The model under review builds one solid part; all positions refer to its coordinate system, in mm. Coordinates: 2 decimals unless noted, no trailing zeros. Put each result on its own line as item: value. Start each with the question number.
Item 1: For pin 1 (0.7 mm diameter, centred on x = -3.87, y = 1.64, fed in from -Z); pin 2 (1.5 mm diameter, centred on x = -3.5, z = 1, fed in from +Y), all flat-tipped, find the tip position at first contact; note any pin that passes through.
Item 2: Consider section A-A on z = 1.65. State how many separate pieces and enclosed holes the cut face has, then the cut area to 3 significant figures.
Item 3: Mouldability with a two-part tool opening along Y and no side actions: class faces 1 (the face through (-23.977, 1.055, 2.972)), 2 (the face through (7.6, 2.3, 2.5)), 3 (the face through (-4.504, 4.555, 2.465)) as pulls with the +Y half, pulls with the -Y half, needs draft (parallel to the pull), parting line crosses it, or undercut.
Item 4: To check wall thickness, follow L1, parallel to X at y = -1.5, z = 3.6; L2, parallel to X at y = -5.5, z = 0.6; L3, parallel to Y at x = -2.5, z = 1.5. State the ranges of each line that lie inside material, in increasing order. Write a range as [from, to].
```python
from build123d import *

# Parameters (mm, degrees)
SCHIZZO1_R                   = 24
SCHIZZO1_R_2                 = 0.6
ESTRUSIONE_ESTRUSIONE1_DEPTH = 5
SMUSSO1_SIZE                 = 1


with BuildPart() as part:
    # Schizzo1 → Estrusione-Estrusione1 (new body)
    with BuildSketch(Plane.XY):
        Circle(SCHIZZO1_R)
        with Locations((-2.2, 0)):
            Circle(SCHIZZO1_R_2, mode=Mode.SUBTRACT)
        Circle(SCHIZZO1_R_2, mode=Mode.SUBTRACT)
        with Locations((-3.866120385, 1.64107074)):
            Circle(SCHIZZO1_R_2, mode=Mode.SUBTRACT)
        with Locations((-1.1, 1.905255888)):
            Circle(SCHIZZO1_R_2, mode=Mode.SUBTRACT)
        with Locations((1.1, 1.905255888)):
            Circle(SCHIZZO1_R_2, mode=Mode.SUBTRACT)
        with Locations((2.2, 0)):
            Circle(SCHIZZO1_R_2, mode=Mode.SUBTRACT)
        with Locations((1.1, -1.905255888)):
            Circle(SCHIZZO1_R_2, mode=Mode.SUBTRACT)
        with Locations((-1.1, -1.905255888)):
            Circle(SCHIZZO1_R_2, mode=Mode.SUBTRACT)
        with Locations((-2.527623097, 3.354269142)):
            Circle(SCHIZZO1_R_2, mode=Mode.SUBTRACT)
        with Locations((-0.511851242, 4.168693837)):
            Circle(SCHIZZO1_R_2, mode=Mode.SUBTRACT)
        with Locations((1.64107074, 3.866120385)):
            Circle(SCHIZZO1_R_2, mode=Mode.SUBTRACT)
        with Locations((3.354269142, 2.527623097)):
            Circle(SCHIZZO1_R_2, mode=Mode.SUBTRACT)
        with Locations((4.168693837, 0.511851242)):
            Circle(SCHIZZO1_R_2, mode=Mode.SUBTRACT)
        with Locations((3.866120385, -1.64107074)):
            Circle(SCHIZZO1_R_2, mode=Mode.SUBTRACT)
        with Locations((2.527623097, -3.354269142)):
            Circle(SCHIZZO1_R_2, mode=Mode.SUBTRACT)
        with Locations((0.511851242, -4.168693837)):
            Circle(SCHIZZO1_R_2, mode=Mode.SUBTRACT)
        with Locations((-1.64107074, -3.866120385)):
            Circle(SCHIZZO1_R_2, mode=Mode.SUBTRACT)
        with Locations((-3.354269142, -2.527623097)):
            Circle(SCHIZZO1_R_2, mode=Mode.SUBTRACT)
        with Locations((-4.168693837, -0.511851242)):
            Circle(SCHIZZO1_R_2, mode=Mode.SUBTRACT)
        with Locations((-6.3, 0)):
            Circle(SCHIZZO1_R_2, mode=Mode.SUBTRACT)
        with Locations((-5.920063511, 2.154726903)):
            Circle(SCHIZZO1_R_2, mode=Mode.SUBTRACT)
        with Locations((-4.826079992, 4.049561941)):
            Circle(SCHIZZO1_R_2, mode=Mode.SUBTRACT)
        with Locations((-3.15, 5.455960044)):
            Circle(SCHIZZO1_R_2, mode=Mode.SUBTRACT)
        with Locations((-1.093983519, 6.204288844)):
            Circle(SCHIZZO1_R_2, mode=Mode.SUBTRACT)
        with Locations((1.093983519, 6.204288844)):
            Circle(SCHIZZO1_R_2, mode=Mode.SUBTRACT)
        with Locations((3.15, 5.455960044)):
            Circle(SCHIZZO1_R_2, mode=Mode.SUBTRACT)
        with Locations((4.826079992, 4.049561941)):
            Circle(SCHIZZO1_R_2, mode=Mode.SUBTRACT)
        with Locations((5.920063511, 2.154726903)):
            Circle(SCHIZZO1_R_2, mode=Mode.SUBTRACT)
        with Locations((6.3, 0)):
            Circle(SCHIZZO1_R_2, mode=Mode.SUBTRACT)
        with Locations((5.920063511, -2.154726903)):
            Circle(SCHIZZO1_R_2, mode=Mode.SUBTRACT)
        with Locations((4.826079992, -4.049561941)):
            Circle(SCHIZZO1_R_2, mode=Mode.SUBTRACT)
        with Locations((3.15, -5.455960044)):
            Circle(SCHIZZO1_R_2, mode=Mode.SUBTRACT)
        with Locations((1.093983519, -6.204288844)):
            Circle(SCHIZZO1_R_2, mode=Mode.SUBTRACT)
        with Locations((-1.093983519, -6.204288844)):
            Circle(SCHIZZO1_R_2, mode=Mode.SUBTRACT)
        with Locations((-3.15, -5.455960044)):
            Circle(SCHIZZO1_R_2, mode=Mode.SUBTRACT)
        with Locations((-4.826079992, -4.049561941)):
            Circle(SCHIZZO1_R_2, mode=Mode.SUBTRACT)
        with Locations((-5.920063511, -2.154726903)):
            Circle(SCHIZZO1_R_2, mode=Mode.SUBTRACT)
        with Locations((-8.448689608, 0.932547001)):
            Circle(SCHIZZO1_R_2, mode=Mode.SUBTRACT)
        with Locations((-7.951343479, 3.004352988)):
            Circle(SCHIZZO1_R_2, mode=Mode.SUBTRACT)
        with Locations((-6.954385197, 4.887384427)):
            Circle(SCHIZZO1_R_2, mode=Mode.SUBTRACT)
        with Locations((-5.520457316, 6.463323528)):
            Circle(SCHIZZO1_R_2, mode=Mode.SUBTRACT)
        with Locations((-3.739658799, 7.633148241)):
            Circle(SCHIZZO1_R_2, mode=Mode.SUBTRACT)
        with Locations((-1.723883767, 8.323354177)):
            Circle(SCHIZZO1_R_2, mode=Mode.SUBTRACT)
        with Locations((0.400209223, 8.49057316)):
            Circle(SCHIZZO1_R_2, mode=Mode.SUBTRACT)
        with Locations((2.499155596, 8.124298204)):
            Circle(SCHIZZO1_R_2, mode=Mode.SUBTRACT)
        with Locations((4.441070831, 7.247543713)):
            Circle(SCHIZZO1_R_2, mode=Mode.SUBTRACT)
        with Locations((6.103937252, 5.915399397)):
            Circle(SCHIZZO1_R_2, mode=Mode.SUBTRACT)
        with Locations((7.383270847, 4.21156878)):
            Circle(SCHIZZO1_R_2, mode=Mode.SUBTRACT)
        with Locations((8.198686382, 2.243109809)):
            Circle(SCHIZZO1_R_2, mode=Mode.SUBTRACT)
        with Locations((8.498948298, 0.133707998)):
            Circle(SCHIZZO1_R_2, mode=Mode.SUBTRACT)
        with Locations((8.265190036, -1.984095178)):
            Circle(SCHIZZO1_R_2, mode=Mode.SUBTRACT)
        with Locations((7.512099486, -3.977230357)):
            Circle(SCHIZZO1_R_2, mode=Mode.SUBTRACT)
        with Locations((6.286996098, -5.720461525)):
            Circle(SCHIZZO1_R_2, mode=Mode.SUBTRACT)
        with Locations((4.666857624, -7.104255057)):
            Circle(SCHIZZO1_R_2, mode=Mode.SUBTRACT)
        with Locations((2.753483321, -8.041662117)):
            Circle(SCHIZZO1_R_2, mode=Mode.SUBTRACT)
        with Locations((0.667097535, -8.47378197)):
            Circle(SCHIZZO1_R_2, mode=Mode.SUBTRACT)
        with Locations((-1.461204443, -8.373462938)):
            Circle(SCHIZZO1_R_2, mode=Mode.SUBTRACT)
        with Locations((-3.497693572, -7.747008434)):
            Circle(SCHIZZO1_R_2, mode=Mode.SUBTRACT)
        with Locations((-5.31440975, -6.633780899)):
            Circle(SCHIZZO1_R_2, mode=Mode.SUBTRACT)
        with Locations((-6.797202018, -5.103728512)):
            Circle(SCHIZZO1_R_2, mode=Mode.SUBTRACT)
        with Locations((-7.852901085, -3.252990093)):
            Circle(SCHIZZO1_R_2, mode=Mode.SUBTRACT)
        with Locations((-8.415173496, -1.197854343)):
            Circle(SCHIZZO1_R_2, mode=Mode.SUBTRACT)
    extrude(amount=ESTRUSIONE_ESTRUSIONE1_DEPTH)

    # Smusso1
    smusso1_edges = [part.edges().sort_by_distance(p)[0] for p in [
        (-24, 0, 0),
    ]]
    chamfer(smusso1_edges, length=SMUSSO1_SIZE)


solid = part.part
```
Report:
1. pin 1: through
1. pin 2: y = 23.84
2. separate pieces: 1
2. enclosed holes: 62
2. area: 1,740 mm²
3. face 1: parting line crosses it
3. face 2: undercut
3. face 3: undercut
4. L1: [-23.95, -8.93], [-7.9, -1.54], [-0.66, 0.66], [1.54, 3.28], [4.45, 7.91], [8.62, 23.95]
4. L2: [-22.95, -7.25], [-6.35, -3.75], [-2.55, 2.55], [3.75, 5.73], [6.85, 22.95]
4. L3: [-23.87, -0.52], [0.52, 2.75], [3.95, 23.87]
